CAD build for the part. Positions are in the model's coordinates, mm. Give positions to 0.01 mm unless a question says otherwise; leave off trailing zeros. Order: outer loops, then holes, each group sorted by start corner. A loop starts at its lowest first (then second) coordinate and runs counter-clockwise, first axis right, second up. Notation, with made-up numbers: (28, -27.5) -> (79, -27.5) arc R8 ccw to (79, -16.5) -> close; hole circle Ø2 at (-13, 87.25). An arc over 180 degrees is marked (long way). Use one line per item in the form item = value. Start each with the question number.
1) Cut at A-A, the plane y = -43. Give the cut face in (x, z), and give its area (3 significant figures).
2) Probe line 1 (X direction, y = -50.5, z = -26); line 2 (Z direction, x = -146.75, y = -76.5); line 3 (Z direction, x = -149.5, y = -90). List the from-to ranges inside material, lowest first.
3) Drop flat-ended pins along their axis: P1, Ø3, axis at y = -63, z = -27.5, coming from the -X side; P2, Ø5, axis at x = -140.5, y = -58.5, coming from the -Z side; P3, Ø1, axis at y = -81, z = -25, coming from the +X side. Give the stop position or say it passes through.
4) Mould opens along X. For faces 1 (the face through (-148.238, -98.389, -26.291)), 2 (the face through (-151.384, -98.389, -25.468)), 3 (the face through (-140, -35.8, -26)) say: pulls with the +X half, pulls with the -X half, needs draft (parallel to the pull), parting line crosses it, or undercut.
from build123d import *

# Parameters (mm, degrees)
SKETCH1_R     = 2
SKETCH1_R_2   = 1.3
CHAMFER1_SIZE = 0.127


with BuildPart() as part:
    # Sweep1: sweep along a curve in space
    with BuildLine() as sweep1_path:
        Line((-150.085279081, -93.282256564, -25.525), (-150.085279081, -103.482256564, -25.525))
        add(Edge.make_bspline(
            [(-138.631112316, -46.6, -27.001603743), (-138.631112316, -53.418290009, -27.001603743), (-144.358195699, -68.791470848, -26.263301872), (-150.085279081, -83.943708487, -25.525), (-150.085279081, -93.282256564, -25.525)],
            knots=[0, 0, 0, 0, 0.425348976, 1, 1, 1, 1], degree=3))
        Line((-138.631112316, -35.8, -27.001603743), (-138.631112316, -46.6, -27.001603743))
    # Sketch1 → Sweep1 (sweep)
    with BuildSketch(Plane(origin=(0, -95.382256564, 0), x_dir=(1, 0, 0), z_dir=(0, 1, 0))):
        with Locations((-150.085279081, 25.525)):
            Circle(SKETCH1_R)
        with Locations((-150.085279081, 25.525)):
            Circle(SKETCH1_R_2, mode=Mode.SUBTRACT)
    sweep(path=sweep1_path.line)

    # Chamfer1
    chamfer1_edges = [part.edges().sort_by_distance(p)[0] for p in [
        (-139.931112316, -35.8, -27.001603743),
        (-140.631112316, -35.8, -27.001603743),
        (-151.385279081, -103.482256564, -25.525),
        (-152.085279081, -103.482256564, -25.525),
    ]]
    chamfer(chamfer1_edges, length=CHAMFER1_SIZE)


solid = part.part
Result:
q1.outline = circle Ø4 at (-138.63, -27); hole circle Ø2.6 at (-138.63, -27)
q1.area = 7.26 mm²
q2.line_1 = -140.65 to -139.76, -138.01 to -137.12
q2.line_2 = -27.89 to -27.18, -24.65 to -23.94
q2.line_3 = -27.49 to -26.76, -24.32 to -23.59
q3.P1 = -144.81
q3.P2 = -28.83
q3.P3 = -146.27
q4.face_1 = parting line crosses it
q4.face_2 = undercut
q4.face_3 = needs draft
